The listing builds one solid part. Answer for the finished solid, in the listing's coordinates (mm). A direction names the side the tool comes from. Coordinates: 2 decimals unless noted, no trailing zeros. Loops run counter-clockwise (first coordinate to the right, second up) from the corner with the lowest first, then second, coordinate; pieces in that order, holes last. Notation, with made-up numbers: M 70.25,-4 L 95.25,-4 A6 cw 95.25,7 Z; hole C -16.5,71.5 d1. An arc over 180 degrees is marked long. Return JSON: item names as keys, results as strings. Group by question number.
1. Section B-B (y = -0.8) is taken. Write down the section's boundary in (x, z), then the cut area to 3 significant figures.
2. The mould has two halves that part along X. Classify faces 4 (the face through (60, 1, -6)), 5 (the face through (55, 1, -12)), 6 (the face through (30, -1, -45.5)), 7 (the face through (4.5, -1, -43)): pulls with the +X half, pulls with the -X half, needs draft (parallel to the pull), parting line crosses it, or undercut.
3. Given P1, Ø1, axis at x = 4.5, y = 0.5, coming from the +Z side; P2, Ø1.5, axis at y = -2, z = -44, coming from the +X side; P3, Ø0.9, axis at y = -1, z = -44.5, coming from the -X side, each flat-ended and moving along its own axis, determine where each tip first touches the part or whether it passes through.
4. Which of the six approach directions +Z, -Z, +X, -X, +Y, -Y give full straight-line access (tool end or side, diameter ignored) to faces 1 (the face through (55, 1, -38)), 2 (the face through (56.721, -1.479, -46.743)), 3 (the face through (57.5, -1, -44))?
5. Section C-C (x = 30) is taken. Write down the section's boundary in (y, z).
6. Straight lines are drawn through the part: L1, parallel to Y at x = 4.5, z = -38.5; L2, parallel to X at y = 1.25, z = -17.5; L3, parallel to Z at x = 33, y = -2.6. For each, find the intervals that lie inside material, in ascending order. Write a range as from..to.
7. Section D-D (x = 24) is taken. Write down the section's boundary in (y, z).
8. Section A-A (z = 4) is taken. Write down the section's boundary in (x, y).
```python
from build123d import *

# Parameters (mm, degrees)
SKETCH1_W           = 60
SKETCH1_H           = 50
BOSS_EXTRUDE1_DEPTH = 2
CHAMFER1_SIZE       = 3
BOSS_EXTRUDE2_DEPTH = 3
SKETCH3_R           = 2
SKETCH3_R_2         = 1.8
BOSS_EXTRUDE3_DEPTH = 2
SKETCH4_W           = 10
SKETCH4_H           = 26
CUT_EXTRUDE1_DEPTH  = 79.262379212
FILLET1_R           = 2


with BuildPart() as part:
    # Sketch1 → Boss-Extrude1 (new body)
    with BuildSketch(Plane(origin=(0, 0, 0), x_dir=(1, 0, 0), z_dir=(0, 1, 0))):
        with Locations((30, 25)):
            Rectangle(SKETCH1_W, SKETCH1_H)
    extrude(amount=BOSS_EXTRUDE1_DEPTH)

    # Chamfer1
    chamfer1_edges = [part.edges().sort_by_distance(p)[0] for p in [
        (0, 1, -50),
        (60, 1, -50),
        (60, 1, 0),
        (0, 1, 0),
    ]]
    chamfer(chamfer1_edges, length=CHAMFER1_SIZE)

    # Sketch2 → Boss-Extrude2 (add)
    with BuildSketch(Plane.XZ):
        Polygon((4.5, -41.5), (2.5, -41.5), (2.5, -45.964466094), (4.035533906, -47.5), (55.964466094, -47.5), (57.5, -45.964466094), (57.5, -41.5), (55.5, -41.5), (55.5, -45.136038969), (55.136038969, -45.5), (4.863961031, -45.5), (4.5, -45.136038969), align=None)
    extrude(amount=BOSS_EXTRUDE2_DEPTH)

    # Sketch3 → Boss-Extrude3 (add)
    # profile 1 of 2: a face of its own
    with BuildSketch(Plane(origin=(0, 2, 0), x_dir=(1, 0, 0), z_dir=(0, 1, 0))):
        with BuildLine():
            Line((18, 0), (26, -8))
            Line((26, -8), (32, -8))
            ThreePointArc((32, -8), (33.414213562, -7.414213562), (34, -6))
            Line((34, -6), (34, 0))
            Line((34, 0), (18, 0))
        make_face()
        with Locations((30, -4)):
            Circle(SKETCH3_R, mode=Mode.SUBTRACT)
    # profile 2 of 2: a face of its own
    with BuildSketch(Plane(origin=(0, 2, 0), x_dir=(1, 0, 0), z_dir=(0, 1, 0))):
        with Locations((30, -4)):
            Circle(SKETCH3_R)
        with Locations(Location((30, -4, 0), (0, 0, 270))):
            Circle(SKETCH3_R_2, mode=Mode.SUBTRACT)
    extrude(amount=-BOSS_EXTRUDE3_DEPTH)

    # Sketch4 → Cut-Extrude1 (cut, through all)
    with BuildSketch(Plane(origin=(0, 2, 0), x_dir=(1, 0, 0), z_dir=(0, 1, 0))):
        with Locations((5, 25)):
            Rectangle(SKETCH4_W, SKETCH4_H)
        with Locations((55, 25)):
            Rectangle(SKETCH4_W, SKETCH4_H)
    extrude(amount=-CUT_EXTRUDE1_DEPTH, mode=Mode.SUBTRACT)

    # Fillet1
    fillet1_edges = [part.edges().sort_by_distance(p)[0] for p in [
        (0, 1, -12),
        (0, 1, -38),
        (10, 1, -38),
        (10, 1, -12),
        (60, 1, -38),
        (60, 1, -12),
        (50, 1, -12),
        (50, 1, -38),
    ]]
    fillet(fillet1_edges, radius=FILLET1_R)


solid = part.part
```
Worked out:
{
 "1": {"outline": "M 2.5,-45.96 L 4.04,-47.5 L 55.96,-47.5 L 57.5,-45.96 L 57.5,-41.5 L 55.5,-41.5 L 55.5,-45.14 L 55.14,-45.5 L 4.86,-45.5 L 4.5,-45.14 L 4.5,-41.5 L 2.5,-41.5 Z", "area": "124 mm^2"},
 "2": {"face 4": "pulls with the +X half", "face 5": "needs draft", "face 6": "undercut", "face 7": "undercut"},
 "3": {"P1": "z = 0", "P2": "x = 57.5", "P3": "x = 2.5"},
 "4": {"face 1": "+X, +Y, -Y", "face 2": "-Z, +X, -Y", "face 3": "+Z, -Z, +X, -Y"},
 "5": {"outline": "M -3,-47.5 L 0,-47.5 L 0,-50 L 2,-50 L 2,2.2 L 0,2.2 L 0,-45.5 L -3,-45.5 Z; M 0,5.8 L 2,5.8 L 2,8 L 0,8 Z"},
 "6": {"L1": "0..2", "L2": "10..50", "L3": "-47.5..-45.5"},
 "7": {"outline": "M -3,-47.5 L 0,-47.5 L 0,-50 L 2,-50 L 2,6 L 0,6 L 0,-45.5 L -3,-45.5 Z"},
 "8": {"outline": "M 22,0 L 28.2,0 L 28.2,2 L 22,2 Z; M 31.8,0 L 34,0 L 34,2 L 31.8,2 Z"}
}
